```python
from build123d import *

# Parameters (mm, degrees)
SKETCH_1_W                            = 54
SKETCH_1_H                            = 48
EXTRUDE_1_DEPTH                       = 5
SKETCH_3_W                            = 3
SKETCH_3_H                            = 8
SKETCH_3_W_2                          = 13
SKETCH_3_H_2                          = 17
SKETCH_3_W_3                          = 5
CUT_EXTRUDE_1_DEPTH                   = 6
CUT_EXTRUDE_2_DEPTH                   = 55
CUT_EXTRUDE_3_DEPTH                   = 6
CUT_EXTRUDE_4_DEPTH                   = 12
HOLE_WIZARD_M31_D                     = 2.5
HOLE_WIZARD_M31_DEPTH                 = 7.5
HOLE_WIZARD_M31_CSINK_D               = 3.2
HOLE_WIZARD_M31_CSINK_ANGLE           = 110
HOLE_WIZARD_M31_TIP                   = 0.751075774
HOLE_WIZARD_M31_ON_FACE_2_D           = 2.5
HOLE_WIZARD_M31_ON_FACE_2_DEPTH       = 7.5
HOLE_WIZARD_M31_ON_FACE_2_CSINK_D     = 3.2
HOLE_WIZARD_M31_ON_FACE_2_CSINK_ANGLE = 110
HOLE_WIZARD_M31_ON_FACE_2_TIP         = 0.751075774


with BuildPart() as part:
    # Эскиз1 → Бобышка-Вытянуть1 (new body)
    with BuildSketch(Plane.XY):
        with Locations((27, 24)):
            Rectangle(SKETCH_1_W, SKETCH_1_H)
    extrude(amount=EXTRUDE_1_DEPTH)

    # Эскиз3 → Вырез-Вытянуть1 (cut, through all)
    with BuildSketch(Plane.XY.offset(5)):
        with Locations((1.5, 44)):
            Rectangle(SKETCH_3_W, SKETCH_3_H)
        with Locations((15.5, 39.5)):
            Rectangle(SKETCH_3_W_2, SKETCH_3_H_2)
        with Locations((51.5, 39.5)):
            Rectangle(SKETCH_3_W_3, SKETCH_3_H_2)
    extrude(amount=-CUT_EXTRUDE_1_DEPTH, mode=Mode.SUBTRACT)

    # Эскиз4 → Вырез-Вытянуть2 (cut, through all)
    with BuildSketch(Plane.ZY):
        Polygon((3.5, 154.254870007), (3.5, 48), (3.5, 46.1), (2.5, 46.1), (2.5, 44.5), (5, 44.5), (111.254870007, 44.5), (262.897242217, 193.3790803), (155.14237221, 303.133950307), align=None)
    extrude(amount=-CUT_EXTRUDE_2_DEPTH, mode=Mode.SUBTRACT)

    # Эскиз5 → Вырез-Вытянуть3 (cut, through all)
    with BuildSketch(Plane.XY.offset(5)):
        with BuildLine():
            Line((48, -145.764501988), (48, 0))
            Line((48, 0), (48, 18))
            ThreePointArc((48, 18), (37, 29), (26, 18))
            Line((26, 18), (0, 18))
            Line((0, 18), (-145.764501988, 18))
            Line((-145.764501988, 18), (-333.948083842, -204.656910244))
            Line((-333.948083842, -204.656910244), (-140.183581854, -368.421412232))
            Line((-140.183581854, -368.421412232), (48, -145.764501988))
        make_face()
    extrude(amount=-CUT_EXTRUDE_3_DEPTH, mode=Mode.SUBTRACT)

    # Эскиз6 → Вырез-Вытянуть4 (cut)
    with BuildSketch(Plane(origin=(0, 48, 0), x_dir=(1, 0, 0), z_dir=(0, 1, 0))):
        with BuildLine():
            ThreePointArc((35.958236434, 0), (49.389746559, 10.032869731), (54.5, 26))
            ThreePointArc((54.5, 26), (4.610253441, 41.967130269), (35.958236434, 0))
        make_face()
    extrude(amount=-CUT_EXTRUDE_4_DEPTH, mode=Mode.SUBTRACT)

    # Отверстие обработанное метчиком M31
    with Locations(Plane(origin=(0, 22, 2.5), x_dir=(0, 0, -1), z_dir=(-1, 0, 0))):
        with Locations((0, 0), (0, -12)):
            CounterSinkHole(HOLE_WIZARD_M31_D / 2, HOLE_WIZARD_M31_CSINK_D / 2, depth=HOLE_WIZARD_M31_DEPTH, counter_sink_angle=HOLE_WIZARD_M31_CSINK_ANGLE)
            with Locations((0, 0, -(HOLE_WIZARD_M31_DEPTH + HOLE_WIZARD_M31_TIP / 2))):  # 118° drill point
                Cone(0, HOLE_WIZARD_M31_D / 2, HOLE_WIZARD_M31_TIP, mode=Mode.SUBTRACT)

    # Отверстие обработанное метчиком M31 on face 2
    with Locations(Plane(origin=(51, 0, 2.5), x_dir=(0, 0, -1), z_dir=(0, -1, 0))):
        with Locations((0, 0)):
            CounterSinkHole(HOLE_WIZARD_M31_ON_FACE_2_D / 2, HOLE_WIZARD_M31_ON_FACE_2_CSINK_D / 2, depth=HOLE_WIZARD_M31_ON_FACE_2_DEPTH, counter_sink_angle=HOLE_WIZARD_M31_ON_FACE_2_CSINK_ANGLE)
            with Locations((0, 0, -(HOLE_WIZARD_M31_ON_FACE_2_DEPTH + HOLE_WIZARD_M31_ON_FACE_2_TIP / 2))):  # 118° drill point
                Cone(0, HOLE_WIZARD_M31_ON_FACE_2_D / 2, HOLE_WIZARD_M31_ON_FACE_2_TIP, mode=Mode.SUBTRACT)

    # Эскиз10 → Вырез-Повернуть1 (revolve, cut)
    with BuildSketch(Plane(origin=(1.455771366, -2.52146997, 0), x_dir=(0, 0, -1), z_dir=(-0.5, 0.866025404, 0))):
        Polygon((-6.082903769, -46.04293994), (2, -60.04293994), (2, -46.04293994), align=None)
    revolve(axis=Axis((41.330127019, 20.5, 5.306460427), (0, 0, -1)), mode=Mode.SUBTRACT)


solid = part.part
```
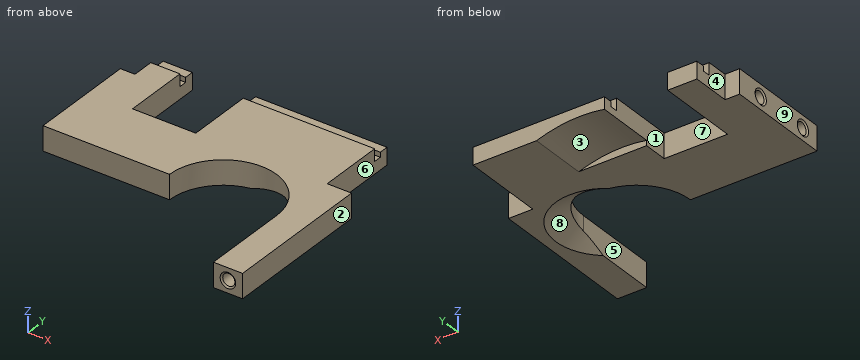
The listing builds one solid part. Answer for the finished solid, in the listing's coordinates (mm). Face numbers are marked on the shaded views. A direction names the side the tool comes from. Round coordinates to 2 decimals unless told otherwise and drop trailing zeros. Write each loop counter-clockwise with the first axis right and the second up, starting at its lowest first coordinate (ties: lowest second). Pieces come first, ordered by that corner, then holes. Notation, with made-up numbers: (84, -23) -> (129, -23) arc R3 ccw to (129, -18) -> close; hole circle Ø2 at (45, -18.5). An arc over 180 degrees is marked (long way). Write item = value, one per line.
1) Given pin 1 (2.5 mm diameter, centred on y = 43, z = 3.5, fed in from -X); pin 2 (1.1 mm diameter, centred on x = 6, z = 3, fed in from -Y); pin 3 (1 mm diameter, centred on x = 30, y = 47, fed in from +Z), each flat-ended and moving along its own axis, determine where each tip first touches the part or whether it passes through.
Check values:
pin_1 = 3
pin_2 = 18
pin_3 = 3.5
2) For a pull along X with two mould halves and no side action, classify the marked faces 6, 7, 8 and 9 as released by +X, released by -X, zero draft, split by the parting line, or undercut.
Check values:
face_6 = released by +X
face_7 = undercut
face_8 = undercut
face_9 = released by -X
3) Straight lines are drawn through the part: line 1 along X through (y, z) = (2, 2.5); line 2 along Y through (x, z) = (2, 2.5); line 3 along Z through (x, y) = (51, 3.5). For each, find the intervals that lie inside material, in ascending order. Write a range as [from, to].
Check values:
line_1 = [48, 49.75], [52.25, 54]
line_2 = [18, 20.75], [23.25, 32.75], [35.25, 40]
line_3 = [0, 1.25], [3.75, 5]
4) Which of the six approach directions +Z, -Z, +X, -X, +Y, -Y give full straight-line access (tool end or side, diameter ignored) to the marked faces 1, 2, 3, 4 and 5?
Check values:
face_1 = +Z, -Z, +Y
face_2 = +Z, -Z, +X, +Y, -Y
face_3 = -Z, +Y
face_4 = +Z, -Z, -X, +Y
face_5 = +Z, -Z, -X, -Y
5) Section A-A on x = 5 is taken. Write down the section's boundary in (y, z).
Check values:
outline = (18, 0) -> (48, 0) -> (48, 3.5) -> (46.1, 3.5) -> (46.1, 2.5) -> (44.5, 2.5) -> (44.5, 5) -> (18, 5) -> close; hole circle Ø2.5 at (22, 2.5); hole circle Ø2.5 at (34, 2.5)
6) Section C-C on x = 18.5 is taken. Write down the section's boundary in (y, z), plus the area to 3 significant figures.
Check values:
outline = (18, 0) -> (31, 0) -> (31, 5) -> (18, 5) -> close
area = 65.0 mm²
7) Section B-B on y = 6.5 is taken. Write down the section's boundary in (x, z), plus the area to 3 significant figures.
Check values:
outline = (48, 0) -> (54, 0) -> (54, 5) -> (48, 5) -> close; hole circle Ø2.5 at (51, 2.5)
area = 25.1 mm²
